from build123d import *

# Parameters (mm, degrees)
BOSS_EXTRUDE1_DEPTH = 12.7
SKETCH2_R           = 4.1021
CUT_EXTRUDE1_DEPTH  = 4.064
SKETCH3_R           = 2.54
CUT_EXTRUDE2_DEPTH  = 85.28690538
SKETCH4_R           = 1.9304
BOSS_EXTRUDE2_DEPTH = 10.16
FILLET1_R           = 1.651
CHAMFER1_SIZE       = 3.81
FILLET2_R           = 1.905
CHAMFER2_SIZE       = 0.635
CHAMFER3_SIZE       = 0.508


with BuildPart() as part:
    # Sketch1 → Boss-Extrude1 (new body)
    with BuildSketch(Plane(origin=(0, 0, 0), x_dir=(1, 0, 0), z_dir=(0, 1, 0))):
        Polygon((0, 0), (0, -4.445), (24.258236459, -4.445), (43.625736459, -15.0975), (82.2325, -15.0975), (82.2325, -9.3825), (70.1675, -9.3825), (70.1675, -10.6525), (44.7675, -10.6525), (25.4, 0), align=None)
    extrude(amount=BOSS_EXTRUDE1_DEPTH)

    # Sketch2 → Cut-Extrude1 (cut)
    with BuildSketch(Plane(origin=(0, 0, 9.3825), x_dir=(-1, 0, 0), z_dir=(0, 0, -1))):
        with Locations((-76.2, 6.35)):
            Circle(SKETCH2_R)
    extrude(amount=-CUT_EXTRUDE1_DEPTH, mode=Mode.SUBTRACT)

    # Sketch3 → Cut-Extrude2 (cut, through all)
    with BuildSketch(Plane(origin=(0, 0, 13.4465), x_dir=(-1, 0, 0), z_dir=(0, 0, -1))):
        with Locations((-76.2, 6.35)):
            Circle(SKETCH3_R)
    extrude(amount=-CUT_EXTRUDE2_DEPTH, mode=Mode.SUBTRACT)

    # Sketch4 → Boss-Extrude2 (add)
    with BuildSketch(Plane(origin=(0, 0, 4.445), x_dir=(-1, 0, 0), z_dir=(0, 0, -1))):
        with Locations((-6.35, 6.35)):
            Circle(SKETCH4_R)
    extrude(amount=-BOSS_EXTRUDE2_DEPTH)

    # Fillet1
    fillet1_edges = [part.edges().sort_by_distance(p)[0] for p in [
        (8.2804, 6.35, 4.445),
    ]]
    fillet(fillet1_edges, radius=FILLET1_R)

    # Chamfer1
    chamfer1_edges = [part.edges().sort_by_distance(p)[0] for p in [
        (82.2325, 0, 12.24),
        (0, 0, 2.2225),
        (82.2325, 12.7, 12.24),
        (0, 12.7, 2.2225),
    ]]
    chamfer(chamfer1_edges, length=CHAMFER1_SIZE)

    # Fillet2
    # the kernel refuses this fillet: 1.905 mm, written as the material it adds along each edge
    with BuildSketch(Plane(origin=(24.258236459, 0, 4.445), x_dir=(-1, 0, 0), z_dir=(0, 1, 0))) as fillet2_piece_1:
        with BuildLine():
            CenterArc((FILLET2_R * 0.256864688635, FILLET2_R), FILLET2_R, 241.188354533, 28.811645467)
            Line((-FILLET2_R * 0.225067086378, FILLET2_R * 0.123791255332), (0, 0))
            Line((0, 0), (FILLET2_R * 0.256864688635, 0))
        make_face()
    extrude(amount=12.7)
    with BuildSketch(Plane(origin=(44.7675, 0, 10.6525), x_dir=(-0.8762087446678116, 0, -0.4819317750134946), z_dir=(0, 1, 0))) as fillet2_piece_2:
        with BuildLine():
            CenterArc((FILLET2_R * 0.256864688635, -FILLET2_R), FILLET2_R, 90, 28.811645467)
            Line((-FILLET2_R * 0.225067086378, -FILLET2_R * 0.123791255332), (0, 0))
            Line((0, 0), (FILLET2_R * 0.256864688635, 0))
        make_face()
    extrude(amount=12.7)
    with BuildSketch(Plane(origin=(70.1675, 0, 10.6525), x_dir=(-1, 0, 0), z_dir=(0, 1, 0))) as fillet2_piece_3:
        with BuildLine():
            CenterArc((1.796051224, -1.905), FILLET2_R, 90, 70.528779366)
            Line((0, -1.27), (0, 0))
            Line((0, 0), (1.796051224, 0))
        make_face()
    extrude(amount=12.7)
    # the kernel refuses this fillet: 1.905 mm, written as the material it takes off along each edge
    with BuildSketch(Plane(origin=(43.625736459, -1.22331808, 15.0975), x_dir=(-0.8762087446678133, 0, -0.4819317750134918), z_dir=(0, 1, 0))) as fillet2_2_piece_1:
        with BuildLine():
            CenterArc((FILLET2_R * 0.256864688635, -FILLET2_R), FILLET2_R, 90, 28.811645467)
            Line((-FILLET2_R * 0.225067086378, -FILLET2_R * 0.123791255332), (0, 0))
            Line((0, 0), (FILLET2_R * 0.256864688635, 0))
        make_face()
    extrude(amount=15.146636159, mode=Mode.SUBTRACT)
    with BuildSketch(Plane(origin=(25.4, -1.22331808, 0), x_dir=(-1, 0, 0), z_dir=(0, 1, 0))) as fillet2_2_piece_2:
        with BuildLine():
            CenterArc((FILLET2_R * 0.256864688635, FILLET2_R), FILLET2_R, 241.188354533, 28.811645467)
            Line((-FILLET2_R * 0.225067086378, FILLET2_R * 0.123791255332), (0, 0))
            Line((0, 0), (FILLET2_R * 0.256864688635, 0))
        make_face()
    extrude(amount=15.146636159, mode=Mode.SUBTRACT)

    # Chamfer2
    chamfer2_edges = [part.edges().sort_by_distance(p)[0] for p in [
        (80.3021, 6.35, 9.3825),
    ]]
    chamfer(chamfer2_edges, length=CHAMFER2_SIZE)

    # Chamfer3
    chamfer3_edges = [part.edges().sort_by_distance(p)[0] for p in [
        (8.2804, 6.35, 14.605),
    ]]
    chamfer(chamfer3_edges, length=CHAMFER3_SIZE)


solid = part.part
Model file for the job. Use its own axes, mm. A direction names the side the tool comes from. Coordinates: 2 decimals unless noted, no trailing zeros. Write each loop counter-clockwise with the first axis right and the second up, starting at its lowest first coordinate (ties: lowest second). Pieces come first, ordered by that corner, then holes. Notation, with made-up numbers: (25, 65.25) -> (38, 65.25) arc R33 cw to (38, 102.25) -> close; hole circle Ø8 at (25.5, 15.25). An arc over 180 degrees is marked (long way). One line per item, written item: value. Start each with the question number.
1) Slice it at B-B on x = 6.35. Write the cut outline in (y, z) (3 decimals).
2) Slice it at D-D on x = 40. Write the cut outline in (y, z).
3) Probe probe 1 along X at (y, z) = (6.5, 10.5); probe 2 along Y at (x, z) = (76.2, 13.8); probe 3 along Y at (x, z) = (76.2, 11.2). List the from-to ranges inside material, lowest first.
4) Flat gauge pins, fed straight in: pin 1 Ø4 at (x, z) = (11.5, 12.5) entering from -Y; pin 2 Ø6 at (x, y) = (73.5, 8.5) entering from -Z; pin 3 Ø6 at (x, y) = (76.2, 6.35) entering from -Z; pin 4 Ø1 at (x, y) = (67, 7.5) entering from -Z. Where does each tip first touch, or does it go through?
5) Pull direction Y, two halves, no side cores. Call faces 1 (the face through (0, 6, 2)), 2 (the face through (41, 0, 9)), 3 (the face through (74, 8, 13.446)): +Y half, -Y half, draft (parallel to the pull), parting line (faces both ways), or undercut.
6) Slice it at C-C on z = 2.5. Write the cut outline in (x, y), then the cut area to 3 significant figures.
7) Which spindle directions (+Z, -Z, +X, -X, +Y, -Y) get a long thin tool onto all of the face, cutting with end or side? Do faces 4 (the face through (69.46, 6.26, 10.31)), 5 (the face through (14, 6, 4.445)), 6 (the face through (72.287, 7.582, 11.708)). Say none if no direction does.
8) Slice it at A-A on x = 76.2. Write the cut outline in (y, z).
Answers follow:
1. outline: (0, 0) -> (12.7, 0) -> (12.7, 4.445) -> (9.931, 4.445) arc R1.651 cw to (8.28, 6.096) -> (8.28, 14.097) -> (7.772, 14.605) -> (4.928, 14.605) -> (4.42, 14.097) -> (4.42, 6.096) arc R1.651 cw to (2.769, 4.445) -> (0, 4.445) -> close
2. outline: (0, 8.03) -> (12.7, 8.03) -> (12.7, 13.1) -> (0, 13.1) -> close
3. probe 1: 4.43 to 8.27, 35.27 to 44.51, 69.12 to 72.1, 80.3 to 82.23
3. probe 2: 0 to 3.81, 8.89 to 12.7
3. probe 3: 0 to 2.25, 10.45 to 12.7
4. pin 1: through
4. pin 2: z = 9.38
4. pin 3: z = 13.45
4. pin 4: z = 10.65
5. face 1: draft
5. face 2: -Y half
5. face 3: undercut
6. outline: (0, 3.81) -> (3.81, 0) -> (29.95, 0) -> (29.95, 12.7) -> (3.81, 12.7) -> (0, 8.89) -> close
6. area: 366 mm2
7. face 4: -Z, +Y, -Y
7. face 5: +Z
7. face 6: -Z
8. outline: (0, 9.38) -> (1.61, 9.38) -> (2.25, 10.02) -> (2.25, 13.45) -> (3.81, 13.45) -> (3.81, 15.1) -> (0, 15.1) -> close; (8.89, 13.45) -> (10.45, 13.45) -> (10.45, 10.02) -> (11.09, 9.38) -> (12.7, 9.38) -> (12.7, 15.1) -> (8.89, 15.1) -> close
